```python
from build123d import *

# Parameters (mm, degrees)
SKETCH1_R           = 2.5
BOSS_EXTRUDE1_DEPTH = 8.6
FILLET1_R           = 2.5
BOSS_EXTRUDE2_DEPTH = 1
SKETCH3_R           = 2.7
BOSS_EXTRUDE3_DEPTH = 1


with BuildPart() as part:
    # Sketch1 → Boss-Extrude1 (new body)
    with BuildSketch(Plane(origin=(0, 0, 0), x_dir=(1, 0, 0), z_dir=(0, 1, 0))):
        Circle(SKETCH1_R)
    extrude(amount=BOSS_EXTRUDE1_DEPTH)

    # Fillet1
    fillet1_edges = [part.edges().sort_by_distance(p)[0] for p in [
        (-2.5, 8.6, 0),
    ]]
    fillet(fillet1_edges, radius=FILLET1_R)

    # Sketch2 → Boss-Extrude2 (add)
    with BuildSketch(Plane(origin=(0, 0, 0), x_dir=(-1, 0, 0), z_dir=(0, -1, 0))):
        Polygon((0, 3), (-3, 3), (-3, -5), (0, -5), (3, -5), (3, 3), align=None)
    extrude(amount=BOSS_EXTRUDE2_DEPTH)

    # Sketch3 → Boss-Extrude3 (add)
    with BuildSketch(Plane(origin=(0, 0, 0), x_dir=(1, 0, 0), z_dir=(0, 1, 0))):
        Circle(SKETCH3_R)
    extrude(amount=BOSS_EXTRUDE3_DEPTH)


solid = part.part
```
Geometry check sheet. Reference: the model listing, model coordinates, mm. A direction names the side the tool comes from. Coordinates: 2 decimals unless noted, no trailing zeros. Order: outer loops, then holes, each group sorted by start corner. A loop starts at its lowest first (then second) coordinate and runs counter-clockwise, first axis right, second up. Notation, with made-up numbers: M 34,9 L 46,9 A22 ccw 46,28 Z; hole C 11,1.25 d3. An arc over 180 degrees is marked long. Answer as a JSON object with one key per item and string values.
Q1. Cross-section at A-A on z = 0. Record the cut outline in (x, y), and give its area (3 significant figures).
Results are:
{"outline": "M -3,-1 L 3,-1 L 3,0 L 2.7,0 L 2.7,1 L 2.5,1 L 2.5,6.1 A2.5 ccw -2.5,6.1 L -2.5,1 L -2.7,1 L -2.7,0 L -3,0 Z", "area": "46.7 mm²"}
Q2. Cross-section at D-D on z = 3. Record the cut outline in (x, y).
Results are:
{"outline": "M -3,-1 L 3,-1 L 3,0 L -3,0 Z"}
Q3. Tool access check on faces 1 (the flat face through (0, -0.5, 5)), 2 (the flat face through (0, 0, 3)). Record the directions out of +Z, -Z, +X, -X, +Y, -Y that give a thin tool (end or side, any length) a straight path to the whole face; none if there is none.
Results are:
{"face 1": "+Z, +X, -X, +Y, -Y", "face 2": "+Y"}
Q4. Depth check by flat-ended pin: pin 1 Ø1 at (y, z) = (2.5, 0) entering from +X; pin 2 Ø1.8 at (x, z) = (1, 2) entering from +Y; pin 3 Ø2 at (y, z) = (4, -2) entering from +X. Enter the tip coordinate at first touch or a pass-through.
Results are:
{"pin 1": "stops at x = 2.5", "pin 2": "stops at y = 8.21", "pin 3": "stops at x = 2.29"}
Q5. Cross-section at C-C on y = 5.5. Record the cut outline in (x, z).
Results are:
{"outline": "C 0,0 d5"}
Q6. Cross-section at B-B on x = 0. Record the cut outline in (y, z).
Results are:
{"outline": "M -1,-3 L 0,-3 L 0,-2.7 L 1,-2.7 L 1,-2.5 L 6.1,-2.5 A2.5 ccw 6.1,2.5 L 1,2.5 L 1,2.7 L 0,2.7 L 0,5 L -1,5 Z"}
Q7. Scan lines: line 1 (Y direction, x = -0.5, z = 3.5); line 2 (Y direction, x = -0.5, z = 2.5); line 3 (X direction, y = 1.5, z = -0.5). Record each from-to range of solid material in increasing order.
Results are:
{"line 1": "y = -1 to 0", "line 2": "y = -1 to 1", "line 3": "x = -2.45 to 2.45"}
